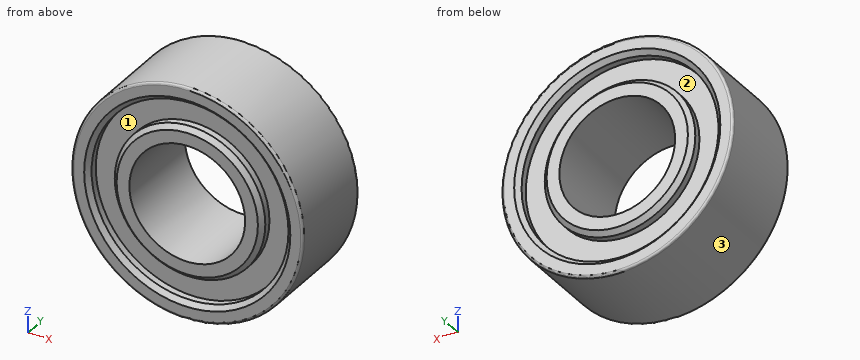
```python
from build123d import *

# Parameters (mm, degrees)
SKETCH2_R           = 5
SKETCH2_R_2         = 2.5
BOSS_EXTRUDE1_DEPTH = 2
SKETCH3_R           = 4.25
SKETCH3_R_2         = 3.25
CUT_EXTRUDE1_DEPTH  = 0.5
CHAMFER1_SIZE       = 0.2
FILLET1_R           = 0.1


with BuildPart() as part:
    # Sketch2 → Boss-Extrude1 (new body, symmetric)
    with BuildSketch(Plane(origin=(0, 0, 0), x_dir=(1, 0, 0), z_dir=(0, 1, 0))):
        Circle(SKETCH2_R)
        Circle(SKETCH2_R_2, mode=Mode.SUBTRACT)
    extrude(amount=BOSS_EXTRUDE1_DEPTH, both=True)

    # Sketch3 → Cut-Extrude1 (cut)
    with BuildSketch(Plane(origin=(0, 2, 0), x_dir=(1, 0, 0), z_dir=(0, 1, 0))):
        Circle(SKETCH3_R)
        Circle(SKETCH3_R_2, mode=Mode.SUBTRACT)
    cut_extrude1 = extrude(amount=-CUT_EXTRUDE1_DEPTH, mode=Mode.SUBTRACT)

    # Mirror1: Cut-Extrude1 across plane
    add(cut_extrude1.mirror(Plane.ZX), mode=Mode.SUBTRACT)

    # Chamfer1
    chamfer1_edges = [part.edges().sort_by_distance(p)[0] for p in [
        (-4.25, 2, 0),
        (-3.25, 2, 0),
        (-3.25, -2, 0),
        (-4.25, -2, 0),
    ]]
    chamfer(chamfer1_edges, length=CHAMFER1_SIZE)

    # Fillet1
    fillet1_edges = [part.edges().sort_by_distance(p)[0] for p in [
        (-5, -2, 0),
        (-5, 2, 0),
    ]]
    fillet(fillet1_edges, radius=FILLET1_R)


solid = part.part
```
Geometry: final body of the model. Coordinates: model frame, mm. Face numbers are marked on the shaded views. Give positions to 0.01 mm unless a question says otherwise; leave off trailing zeros. Loops run counter-clockwise (first coordinate to the right, second up) from the corner with the lowest first, then second, coordinate; pieces in that order, holes last. Notation, with made-up numbers: (-15.75, 68) - (20.25, 68) arc R23 ccw to (20.25, 84) - close; hole circle Ø6 at (84, 9.5). An arc over 180 degrees is marked (long way). Answer as CSV lines item,"result". Start each with the question number.
(1) Ray query, line 1 along X through (y, z) = (1.6, 0); line 2 along X through (y, z) = (0, 0). Return the intervals inside material, ascending. Write a range as [from, to].
(2) Mould query, pull axis Z, two halves, no side actions, for the marked faces 1, 2 and 3. Classes: +Z half, -Z half, draft (parallel to the pull), parting line (faces both ways), or undercut.
(3) Section query A-A (y = -1.3). Output: boundary loops of the cut face in (x, z), and give its area (3 significant figures).
(4) Pin query (flat end, axial travel): P1, Ø2, axis at y = -1.5, z = 3.5, coming from the +X side. Return the tip coordinate at first contact, or that it passes through.
Worked answers:
1,line 1,"x = [-5, -4.25], [-3.25, -2.5], [2.5, 3.25], [4.25, 5]"
1,line 2,"x = [-5, -2.5], [2.5, 5]"
2,face 1,"undercut"
2,face 2,"undercut"
2,face 3,"parting line"
3,outline,"circle Ø10 at (0, 0); hole circle Ø5 at (0, 0)"
3,area,"58.9 mm^2"
4,P1,"stops at x = 4.33"
